Check sheet for the modelled part. Datum: model origin and axes. Units: mm. A direction names the side the tool comes from. Give positions to 0.01 mm unless a question says otherwise; leave off trailing zeros. Write each loop counter-clockwise with the first axis right and the second up, starting at its lowest first coordinate (ties: lowest second). Pieces come first, ordered by that corner, then holes. Notation, with made-up numbers: M -23,48.5 L -3,48.5 A16 cw -3,77.5 Z; hole C 68,5.25 d3. An arc over 180 degrees is marked long. Use CSV: the item, a comma, the result in double quotes. Start each with the question number.
1. Cross-section at A-A, the plane x = 0. Enter the section's corners in (y, z).
2. Access from +Z, -Z, +X, -X, +Y, -Y to the whole of each face (thin tool, end or side, straight path). Record for faces 1 (the face through (-0.65, 76.05, 141.48)), 2 (the face through (-0.65, -73.95, 141.48)), 3 (the face through (-1.08, -4.88, 72.19)).
3. Cross-section at C-C, the plane z = 227.5. Enter the section's corners in (x, y).
4. Depth check by flat-ended pin: P1, Ø3, axis at x = -1.5, z = 184.5, coming from the +Y side; P2, Ø1.5, axis at x = -1.5, z = 125.5, coming from the +Y side; P3, Ø1, axis at x = -3, z = 110, coming from the -Y side. Enter the tip coordinate at first touch or a pass-through.
5. Cross-section at B-B, the plane y = 15. Enter the section's corners in (x, z).
6. Scan lines: line 1 (Y direction, x = -0.25, z = 127.5); line 2 (Y direction, x = -3.5, z = 257.5); line 3 (Z direction, x = 4.5, y = -30.5). Record each from-to range of solid material in increasing order.
from build123d import *

# Parameters (mm, degrees)
SKETCH1_R           = 5
BOSS_EXTRUDE1_DEPTH = 300
SKETCH2_R           = 5
BOSS_EXTRUDE2_DEPTH = 150


with BuildPart() as part:
    # Sketch1 → Boss-Extrude1 (new body)
    with BuildSketch(Plane.XY):
        Circle(SKETCH1_R)
    extrude(amount=BOSS_EXTRUDE1_DEPTH)

    # Sketch2 → Boss-Extrude2 (add, symmetric)
    with BuildSketch(Plane(origin=(0, 0, 0), x_dir=(1, 0, 0), z_dir=(0, 1, 0))):
        with Locations((0, -146.435568709)):
            Circle(SKETCH2_R)
    extrude(amount=BOSS_EXTRUDE2_DEPTH, both=True)


solid = part.part
Worked answers:
1,outline,"M -150,141.44 L -5,141.44 L -5,0 L 5,0 L 5,141.44 L 150,141.44 L 150,151.44 L 5,151.44 L 5,300 L -5,300 L -5,151.44 L -150,151.44 Z"
2,face 1,"+Y"
2,face 2,"-Y"
2,face 3,"-Z"
3,outline,"C 0,0 d10"
4,P1,"stops at y = 5"
4,P2,"stops at y = 4.94"
4,P3,"stops at y = -4.33"
5,outline,"C 0,146.44 d10"
6,line 1,"y = -4.99 to 4.99"
6,line 2,"y = -3.57 to 3.57"
6,line 3,"z = 144.26 to 148.62"
